Verification items for the finished model (mm, model axes). A direction names the side the tool comes from. Round coordinates to 2 decimals unless told otherwise and drop trailing zeros. Write each loop counter-clockwise with the first axis right and the second up, starting at its lowest first coordinate (ties: lowest second). Pieces come first, ordered by that corner, then holes. Notation, with made-up numbers: M 71,73 L 119,73 A30 ccw 119,101 Z; hole C 47,65.5 d2. An arc over 180 degrees is marked long. Use a Markdown table: item, result. Add a question column.
from build123d import *

# Parameters (mm, degrees)
SKETCH_1_W          = 40
SKETCH_1_H          = 20
SKETCH_1_W_2        = 36
SKETCH_1_H_2        = 16
EXTRUDE_1_DEPTH     = 50
SKETCH_2_R          = 1.5
CUT_EXTRUDE_1_DEPTH = 50
SKETCH_3_R          = 1.5
CUT_EXTRUDE_2_DEPTH = 50


with BuildPart() as part:
    # 草图1 → 凸台-拉伸1 (new body)
    with BuildSketch(Plane.XY):
        Rectangle(SKETCH_1_W, SKETCH_1_H)
        Rectangle(SKETCH_1_W_2, SKETCH_1_H_2, mode=Mode.SUBTRACT)
    extrude(amount=EXTRUDE_1_DEPTH)

    # 草图2 → 切除-拉伸1 (cut)
    with BuildSketch(Plane(origin=(0, 10, 0), x_dir=(1, 0, 0), z_dir=(0, 1, 0))):
        with Locations(Location((-15, -20, 0), (0, 0, 270))):
            Circle(SKETCH_2_R)
        with Locations(Location((15, -2.679491924, 0), (0, 0, 270))):
            Circle(SKETCH_2_R)
        with Locations(Location((15, -37.320508076, 0), (0, 0, 270))):
            Circle(SKETCH_2_R)
    extrude(amount=-CUT_EXTRUDE_1_DEPTH, mode=Mode.SUBTRACT)

    # 草图3 → 切除-拉伸2 (cut)
    with BuildSketch(Plane.ZY.offset(20)):
        with Locations(Location((10, 0, 0), (0, 0, 270))):
            Circle(SKETCH_3_R)
        with Locations(Location((30, 0, 0), (0, 0, 270))):
            Circle(SKETCH_3_R)
        with Locations(Location((45, 0, 0), (0, 0, 270))):
            Circle(SKETCH_3_R)
    extrude(amount=-CUT_EXTRUDE_2_DEPTH, mode=Mode.SUBTRACT)


solid = part.part
1. Scan lines: line 1 along Z through (x, y) = (19.4, 0); line 2 along X through (y, z) = (-7, 16.5); line 3 along Y through (x, z) = (-6, 35.5). Record each from-to range of solid material in increasing order. Write a range as from..to.
2. Cross-section at A-A on y = 6.5. Enter the section's corners in (x, z).
3. Cross-section at D-D on x = -2. Enter the section's corners in (y, z).
4. Release check for a two-part mould opening along Z. For faces 1 (the flat face through (-20, 0, 25)), 2 (the cylindrical face through (-14.93, 9.01, 18.5)), 3 (the flat face through (-0.1, 8.2, 50)) record: +Z half, -Z half, draft (parallel to the pull), parting line (faces both ways), or undercut.
5. Cross-section at B-B on z = 24. Enter the section's corners in (x, y).
6. Access from +Z, -Z, +X, -X, +Y, -Y to the whole of each face (thin tool, end or side, straight path). Record for faces 4 (the cylindrical face through (-14.93, -8.99, 18.5)), 5 (the flat face through (0, -8, 25)).
7. Cross-section at C-C on y = 0. Count the separate pieces of the cut face and the enclosed holes in it, plus the area to 3 significant figures.
Answer:
| question | item | result |
|---|---|---|
| 1 | line 1 | z = 0..8.5, 11.5..28.5, 31.5..43.5, 46.5..50 |
| 1 | line 2 | x = -20..-18, 18..20 |
| 1 | line 3 | y = -10..-8, 8..10 |
| 2 | outline | M -20,0 L -18,0 L -18,50 L -20,50 Z; M 18,0 L 20,0 L 20,50 L 18,50 Z |
| 3 | outline | M -10,0 L -8,0 L -8,50 L -10,50 Z; M 8,0 L 10,0 L 10,50 L 8,50 Z |
| 4 | face 1 | draft |
| 4 | face 2 | undercut |
| 4 | face 3 | +Z half |
| 5 | outline | M -20,-10 L 20,-10 L 20,10 L -20,10 Z; hole M -18,-8 L 18,-8 L 18,8 L -18,8 Z |
| 6 | face 4 | +Y, -Y |
| 6 | face 5 | +Z, -Z |
| 7 | separate pieces | 8 |
| 7 | enclosed holes | 0 |
| 7 | area | 164 mm^2 |
